Drawing for the job (mm, zero at the part's lowest x, y, z). Coordinates: 2 decimals unless noted, no trailing zeros. Order: outer loops, then holes, each group sorted by start corner. A loop starts at its lowest first (then second) coordinate and runs counter-clockwise, first axis right, second up. Notation, with made-up numbers: (17, 72) -> (46, 72) arc R29 cw to (46, 110) -> close; hole circle Ø11 at (89.5, 53). An arc over 180 degrees is marked (long way). Write each question's results on one line, items separated by ' | '.
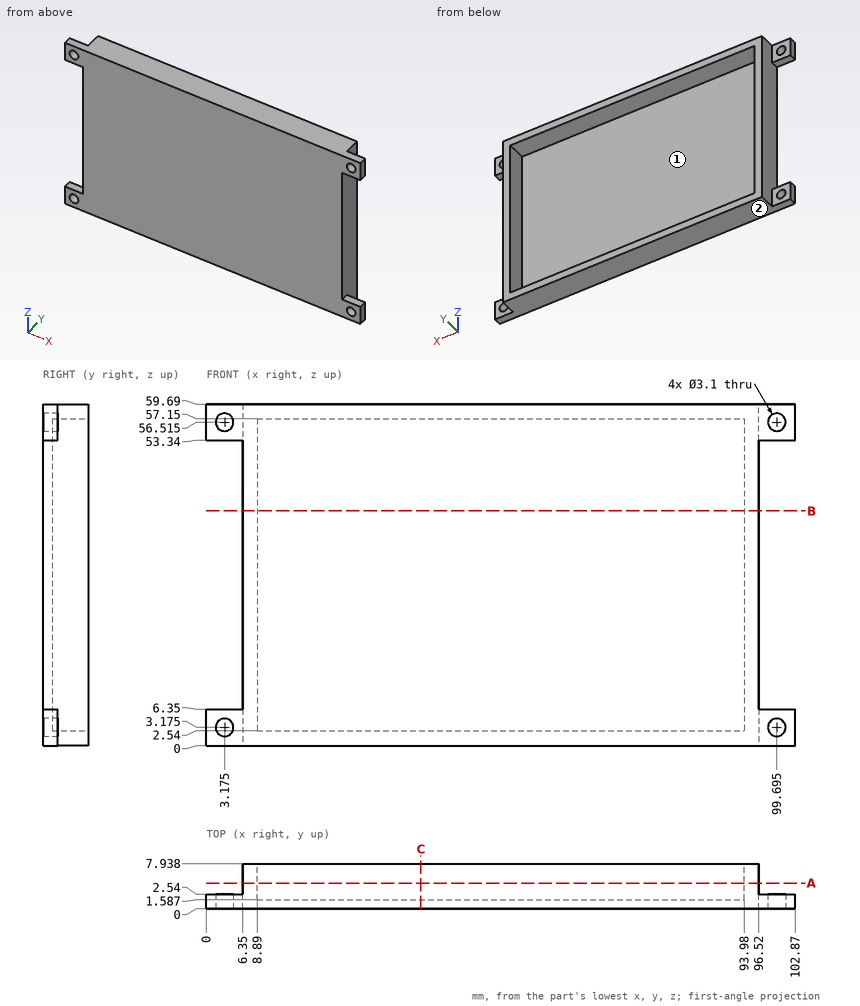
Item 1: Slice it at C-C, the plane x = 37.5. List the corners of the cut face in (y, z), and give its area (3 significant figures).
Answer:
outline: (0, 0) -> (7.94, 0) -> (7.94, 2.54) -> (1.59, 2.54) -> (1.59, 57.15) -> (7.94, 57.15) -> (7.94, 59.69) -> (0, 59.69) -> close | area: 127 mm^2
Item 2: Drill centre lines: line 1 (Z direction, x = 87.5, y = 2.75); line 2 (X direction, y = 6.75, z = 37); line 3 (Y direction, x = 81, z = 55). Where is each one in solid material? Low to high. Write a range as from..to.
Answer:
line 1: z = 0..2.54, 57.15..59.69 | line 2: x = 6.35..8.89, 93.98..96.52 | line 3: y = 0..1.59
Item 3: Pull direction X, two halves, no side cores. Call the marked faces 1 and 2: released by +X, released by -X, zero draft, split by the parting line, or undercut.
Answer:
face 1: undercut | face 2: zero draft
Item 4: Slice it at A-A, the plane y = 4.5. List the corners of the cut face in (x, z).
Answer:
outline: (6.35, 0) -> (96.52, 0) -> (96.52, 59.69) -> (6.35, 59.69) -> close; hole (8.89, 2.54) -> (93.98, 2.54) -> (93.98, 57.15) -> (8.89, 57.15) -> close
Item 5: Pin check, flat tips, straight feed: pin 1 (3 mm diameter, centred on y = 5.5, z = 41, fed in from +X); pin 2 (3 mm diameter, centred on y = 5, z = 48, fed in from -X); pin 3 (5 mm diameter, centred on x = 3.175, z = 3.175, fed in from +Y); pin 4 (4 mm diameter, centred on x = 99.695, z = 56.515, fed in from -Y). Stop position of each tip, or through.
Answer:
pin 1: stops at x = 96.52 | pin 2: stops at x = 6.35 | pin 3: stops at y = 2.54 | pin 4: stops at y = 0
Item 6: Slice it at B-B, the plane z = 41. List the corners of the cut face in (x, y).
Answer:
outline: (6.35, 0) -> (96.52, 0) -> (96.52, 7.94) -> (93.98, 7.94) -> (93.98, 1.59) -> (8.89, 1.59) -> (8.89, 7.94) -> (6.35, 7.94) -> close
